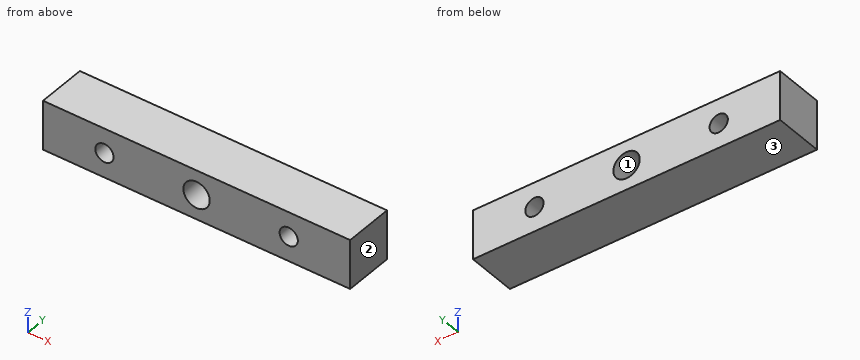
from build123d import *

# Parameters (mm, degrees)
SKETCH1_W           = 50
SKETCH1_H           = 8
BOSS_EXTRUDE1_DEPTH = 8
SKETCH2_R           = 2.145
SKETCH2_R_2         = 1.485
CUT_EXTRUDE1_DEPTH  = 8


with BuildPart() as part:
    # Sketch1 → Boss-Extrude1 (new body)
    with BuildSketch(Plane(origin=(0, 0, 0), x_dir=(1, 0, 0), z_dir=(0, 1, 0))):
        Rectangle(SKETCH1_W, SKETCH1_H)
    extrude(amount=BOSS_EXTRUDE1_DEPTH)

    # Sketch2 → Cut-Extrude1 (cut)
    with BuildSketch(Plane(origin=(0, 8, 0), x_dir=(1, 0, 0), z_dir=(0, 1, 0))):
        with Locations(Location((0, 0, 0), (0, 0, 270))):
            Circle(SKETCH2_R)
        with Locations(Location((-15, 0, 0), (0, 0, 270))):
            Circle(SKETCH2_R_2)
        with Locations(Location((15, 0, 0), (0, 0, 270))):
            Circle(SKETCH2_R_2)
    extrude(amount=-CUT_EXTRUDE1_DEPTH, mode=Mode.SUBTRACT)


solid = part.part
Input: part model. Units: mm. Frame: model coordinates. Face numbers are marked on the shaded views. Round coordinates to 2 decimals unless told otherwise and drop trailing zeros. Loops run counter-clockwise (first coordinate to the right, second up) from the corner with the lowest first, then second, coordinate; pieces in that order, holes last. Notation, with made-up numbers: (86, 25) -> (120, 25) arc R22 cw to (120, 35) -> close; hole circle Ø6 at (-31, 33.5). An arc over 180 degrees is marked (long way). Answer as a JSON object with one key per item and string values. Group by question number.
1) Draft query along X for the marked faces 1, 2 and 3. Return one class per face: +X half, -X half, draft (parallel to the pull), parting line (faces both ways), or undercut.
2) Pin query (flat end, axial travel): pin 1 (4 mm diameter, centred on x = 0, z = 0, fed in from +Y). Return the tip coordinate at first contact, or that it passes through.
3) Section query B-B on z = 0. Output: boundary loops of the cut face in (x, y) (3 decimals).
4) Section query C-C on y = 2.75. Output: boundary loops of the cut face in (x, z) (3 decimals), plus the area to 3 significant figures.
5) Ray query, L1, parallel to X at y = 3.75, z = 0 (3 decimals); L2, parallel to X at y = 3, z = -1; L3, parallel to Z at x = -15.5, y = 7. Return the intervals inside material, ascending.
6) Section query D-D on x = -15. Output: boundary loops of the cut face in (y, z) (3 decimals).
7) Section query A-A on x = 0. Output: boundary loops of the cut face in (y, z) (3 decimals).
Reply:
{
 "1": {"face 1": "undercut", "face 2": "+X half", "face 3": "draft"},
 "2": {"pin 1": "passes through"},
 "3": {"outline": "(-25, 0) -> (-16.485, 0) -> (-16.485, 8) -> (-25, 8) -> close; (-13.515, 0) -> (-2.145, 0) -> (-2.145, 8) -> (-13.515, 8) -> close; (2.145, 0) -> (13.515, 0) -> (13.515, 8) -> (2.145, 8) -> close; (16.485, 0) -> (25, 0) -> (25, 8) -> (16.485, 8) -> close"},
 "4": {"outline": "(-25, -4) -> (25, -4) -> (25, 4) -> (-25, 4) -> close; hole circle Ø2.97 at (-15, 0); hole circle Ø4.29 at (0, 0); hole circle Ø2.97 at (15, 0)", "area": "372 mm2"},
 "5": {"L1": "x = -25 to -16.485, -13.515 to -2.145, 2.145 to 13.515, 16.485 to 25", "L2": "x = -25 to -16.1, -13.9 to -1.9, 1.9 to 13.9, 16.1 to 25", "L3": "z = -4 to -1.4, 1.4 to 4"},
 "6": {"outline": "(0, -4) -> (8, -4) -> (8, -1.485) -> (0, -1.485) -> close; (0, 1.485) -> (8, 1.485) -> (8, 4) -> (0, 4) -> close"},
 "7": {"outline": "(0, -4) -> (8, -4) -> (8, -2.145) -> (0, -2.145) -> close; (0, 2.145) -> (8, 2.145) -> (8, 4) -> (0, 4) -> close"}
}
